```python
from build123d import *

# Parameters (mm, degrees)
F0_W      = 25.4
F0_H      = 25.4
F1_DEPTH  = 12.7
F7_R      = 2.6
F8_DEPTH  = 1.2
F6_R      = 2.6
F9_DEPTH  = 1.2
F5_R      = 2.6
F10_DEPTH = 1.2
F4_R      = 2.6
F11_DEPTH = 1.2
F2_R      = 2.5
F12_DEPTH = 1.2
F3_R      = 2.6
F13_DEPTH = 1.2


with BuildPart() as f1:
    # F0 (on Top) → F1 (new body, symmetric)
    with BuildSketch(Plane.XY):
        Rectangle(F0_W, F0_H)
    extrude(amount=F1_DEPTH, both=True)

    # F7 (on face) → F8 (cut)
    with BuildSketch(Plane(origin=(0, 12.7, 0), x_dir=(-1, 0, 0), z_dir=(0, 1, 0))):
        Circle(F7_R)
    extrude(amount=-F8_DEPTH, mode=Mode.SUBTRACT)

    # F6 (on face) → F9 (cut)
    with BuildSketch(Plane(origin=(0, 0, -12.7), x_dir=(1, 0, 0), z_dir=(0, 0, -1))):
        Circle(F6_R)
    extrude(amount=-F9_DEPTH, mode=Mode.SUBTRACT)

    # F5 (on face) → F10 (cut)
    with BuildSketch(Plane(origin=(-12.7, 0, 0), x_dir=(0, -1, 0), z_dir=(-1, 0, 0))):
        Circle(F5_R)
    extrude(amount=-F10_DEPTH, mode=Mode.SUBTRACT)

    # F4 (on face) → F11 (cut)
    with BuildSketch(Plane.XY.offset(12.7)):
        Circle(F4_R)
    extrude(amount=-F11_DEPTH, mode=Mode.SUBTRACT)

    # F2 (on face) → F12 (cut)
    with BuildSketch(Plane.XZ.offset(12.7)):
        Circle(F2_R)
    extrude(amount=-F12_DEPTH, mode=Mode.SUBTRACT)

    # F3 (on face) → F13 (cut)
    with BuildSketch(Plane.YZ.offset(12.7)):
        Circle(F3_R)
    extrude(amount=-F13_DEPTH, mode=Mode.SUBTRACT)


solid = f1.part
```
Part model, mm, in its own coordinate system. A direction names the side the tool comes from. Give positions to 0.01 mm unless a question says otherwise; leave off trailing zeros. Order: outer loops, then holes, each group sorted by start corner. A loop starts at its lowest first (then second) coordinate and runs counter-clockwise, first axis right, second up. Notation, with made-up numbers: M 18.5,46 L 45.5,46 A35 cw 45.5,81 Z; hole C 88,-13 d3. An arc over 180 degrees is marked long. Use a Markdown table: item, result. Add a question column.
(1) Saw through at B-B, the plane x = 0. Give the cut face in (y, z), and give its area (3 significant figures).
(2) Mould opens along Y. For faces 1 (the face through (3, 12.7, 0)), 2 (the face through (3, -12.7, 0)), 3 (the face through (-11.5, 0, 0)) say: +Y half, -Y half, draft (parallel to the pull), parting line (faces both ways), or undercut.
(3) Saw through at A-A, the plane z = 0. Give the cut face in (x, y).
(4) Probe line 1 along Z through (x, y) = (0, -11.9); line 2 along Y through (x, z) = (0, -12.15). List the from-to ranges inside material, lowest first. Write a range as [from, to].
(5) 3-axis set-ups, long thin cutter, end or side, ignore diameter. For faces 4 (the face through (0, -11.5, 0)), 5 (the face through (0, 0, -11.5)), 6 (the face through (0, 11.5, 0)), 7 (the face through (0, 0, 11.5)): which of +Z, -Z, +X, -X, +Y, -Y reach the whole face in a straight line?
(6) Drop flat-ended pins along their axis: P1, Ø2.5, axis at x = 0, y = 1, coming from the +Z side; P2, Ø2.5, axis at y = -0.5, z = -0.5, coming from the +X side; P3, Ø3, axis at y = 0, z = 0, coming from the -X side. Give the stop position or say it passes through.
Answer key:
| question | item | result |
|---|---|---|
| 1 | outline | M -12.7,-12.7 L -2.6,-12.7 L -2.6,-11.5 L 2.6,-11.5 L 2.6,-12.7 L 12.7,-12.7 L 12.7,-2.6 L 11.5,-2.6 L 11.5,2.6 L 12.7,2.6 L 12.7,12.7 L 2.6,12.7 L 2.6,11.5 L -2.6,11.5 L -2.6,12.7 L -12.7,12.7 L -12.7,2.5 L -11.5,2.5 L -11.5,-2.5 L -12.7,-2.5 Z |
| 1 | area | 620 mm^2 |
| 2 | face 1 | +Y half |
| 2 | face 2 | -Y half |
| 2 | face 3 | undercut |
| 3 | outline | M -12.7,-12.7 L -2.5,-12.7 L -2.5,-11.5 L 2.5,-11.5 L 2.5,-12.7 L 12.7,-12.7 L 12.7,-2.6 L 11.5,-2.6 L 11.5,2.6 L 12.7,2.6 L 12.7,12.7 L 2.6,12.7 L 2.6,11.5 L -2.6,11.5 L -2.6,12.7 L -12.7,12.7 L -12.7,2.6 L -11.5,2.6 L -11.5,-2.6 L -12.7,-2.6 Z |
| 4 | line 1 | [-12.7, -2.5], [2.5, 12.7] |
| 4 | line 2 | [-12.7, -2.6], [2.6, 12.7] |
| 5 | face 4 | -Y |
| 5 | face 5 | -Z |
| 5 | face 6 | +Y |
| 5 | face 7 | +Z |
| 6 | P1 | z = 11.5 |
| 6 | P2 | x = 11.5 |
| 6 | P3 | x = -11.5 |
